```python
from build123d import *

# Parameters (mm, degrees)
F0_W     = 88.3264541626
F0_H     = 62.5167712569
F1_DEPTH = 76.2
F3_DEPTH = 76.201
F4_R     = 12.6699231952
F5_DEPTH = 58.1391964974
F6_W     = 99.7974202037
F6_H     = 75.3260236233
F7_DEPTH = 25.4
F9_DEPTH = 25.401


with BuildPart() as f1:
    # F0 (on Front) → F1 (new body)
    with BuildSketch(Plane.XZ):
        Rectangle(F0_W, F0_H)
    extrude(amount=F1_DEPTH)

    # F2 (on face) → F3 (cut, through all)
    with BuildSketch(Plane.XZ.offset(76.2)):
        Polygon((44.1632270813, 31.2583856285), (-27.3391399533, 31.2583856285), (44.1632270813, -31.2583856285), align=None)
    extrude(amount=-F3_DEPTH, mode=Mode.SUBTRACT)

    # F4 (on face) → F5 (cut, through all)
    with BuildSketch(Plane(origin=(3.6445426056, 0, 4.1683762265), x_dir=(0.752826049, 0, -0.6582195227), z_dir=(0.6582195227, 0, 0.752826049))):
        with Locations((-5.3561865352, -46.0435785353)):
            Circle(F4_R)
    extrude(amount=-F5_DEPTH, mode=Mode.SUBTRACT)

    # F6 (on Front) → F7 (join)
    with BuildSketch(Plane.XZ):
        with Locations((6.1178505421, 6.7869918421)):
            Rectangle(F6_W, F6_H)
    extrude(amount=F7_DEPTH)

    # F8 (on face) → F9 (cut, through all)
    with BuildSketch(Plane.XZ.offset(25.4)):
        Polygon((56.0165606439, 44.4500036538), (-20.7964573056, 44.4500036538), (56.0165606439, -11.8411714114), align=None)
    extrude(amount=-F9_DEPTH, mode=Mode.SUBTRACT)


solid = f1.part
```
Design review of the part built by this model. Coordinates are the model's own, in mm. A direction names the side the tool comes from. Coordinates: 2 decimals unless noted, no trailing zeros. Order: outer loops, then holes, each group sorted by start corner. A loop starts at its lowest first (then second) coordinate and runs counter-clockwise, first axis right, second up. Notation, with made-up numbers: (58, -30) - (115, -30) arc R34 cw to (115, 0) - close; hole circle Ø11 at (-26.75, 12.25). An arc over 180 degrees is marked (long way). One line per question, with ' | ' between items.
Q1. Consider section D-D, the plane x = 36. Give the boundary of the cut face in (y, z).
Answer key:
outline: (-76.2, -31.26) - (0, -31.26) - (0, 2.83) - (-25.4, 2.83) - (-25.4, -24.12) - (-76.2, -24.12) - close
Q2. For faces 4 (the flat face through (-1, -38, -31.258)), 5 (the flat face through (-43.781, -13, 38)), list the 3-axis set-ups (+Z, -Z, +X, -X, +Y, -Y) from which the entire face can be reached by the end or side of a thin tool; tool diameter is ignored.
Answer key:
face 4: -Z, +X, -X, +Y, -Y | face 5: +Z, -X, +Y, -Y
Q3. Clearance check with flat-ended pins moving along their axes: pin 1 Ø5 at (x, z) = (-21.5, 7.5) entering from +Y; pin 2 Ø13.5 at (x, y) = (-33.5, -55.5) entering from +Z; pin 3 Ø10 at (x, y) = (50.5, -17.5) entering from -Z; pin 4 Ø6.5 at (y, z) = (-10, 38.5) entering from -X. State where each tip first meets the part, or that it passes through.
Answer key:
pin 1: stops at y = 0 | pin 2: stops at z = 31.26 | pin 3: stops at z = -30.88 | pin 4: stops at x = -43.78
Q4. Consider section B-B, the plane y = -9.5. Give the boundary of the cut face in (x, z), then the cut area to 3 significant figures.
Answer key:
outline: (-44.16, -31.26) - (44.16, -31.26) - (43.73, -30.88) - (56.02, -30.88) - (56.02, -11.84) - (-20.8, 44.45) - (-43.78, 44.45) - (-43.78, 31.26) - (-44.16, 31.26) - close | area: 5,410 mm2
Q5. Consider section A-A, the plane y = -48. Give the boundary of the cut face in (x, z).
Answer key:
outline: (-44.16, -23.36) - (-9.81, 15.93) - (-27.34, 31.26) - (-44.16, 31.26) - close; (-17.82, -31.26) - (44.16, -31.26) - (9.04, -0.55) - close
Q6. To check wall thickness, follow line 1 along X through (y, z) = (-57, -12.5); line 2 along Y through (x, z) = (-14.5, 37.5); line 3 along Z through (x, y) = (-9, -56). State the ranges of each line that lie inside material, in increasing order.
Answer key:
line 1: x = -44.16 to -26.5, -9.59 to 22.71 | line 2: y = -25.4 to 0 | line 3: z = -31.26 to -14.06, 9.75 to 15.22
Q7. Consider section C-C, the plane z = 27.5. Give the boundary of the cut face in (x, y).
Answer key:
outline: (-44.16, -76.2) - (-23.04, -76.2) - (-23.04, -25.4) - (2.33, -25.4) - (2.33, 0) - (-44.16, 0) - close
Q8. The part is to be moulded in two halves that separate along Z. For faces 1 (the cylindrical face through (-24.53, -45.49, -0.69)), 2 (the flat face through (10, -25.4, 7)), 3 (the flat face through (-32, -13, 44.45)), say which applies: +Z half, -Z half, draft (parallel to the pull), parting line (faces both ways), or undercut.
Answer key:
face 1: undercut | face 2: draft | face 3: +Z half
